Check sheet for the modelled part. Datum: model origin and axes. Units: mm. Face numbers are marked on the shaded views. A direction names the side the tool comes from. Give positions to 0.01 mm unless a question says otherwise; leave off trailing zeros. Order: outer loops, then holes, each group sorted by start corner. A loop starts at its lowest first (then second) coordinate and runs counter-clockwise, first axis right, second up.
from build123d import *

# Parameters (mm, degrees)
F0_R      = 100
F1_DEPTH  = 50
F2_R      = 10
F1_FACE_R = 90
F3_DEPTH  = 3
F5_DEPTH  = 3
F7_W      = 2.681116
F7_H      = 11.75565
F7_W_2    = 14
F7_H_2    = 14
F8_DEPTH  = 3


with BuildPart() as f1:
    # F0 (on Top) → F1 (new body)
    with BuildSketch(Plane.XY):
        Circle(F0_R)
    extrude(amount=F1_DEPTH)

    # F2
    f2_edges = [f1.edges().sort_by_distance(p)[0] for p in [
        (-100, 0, 50),
    ]]
    fillet(f2_edges, radius=F2_R)

    # F1_face (on face) → F3 (cut)
    with BuildSketch(Plane.XY.offset(50)):
        Circle(F1_FACE_R)
    extrude(amount=-F3_DEPTH, mode=Mode.SUBTRACT)

    # F4 (on face) → F5 (join)
    with BuildSketch(Plane.XY.offset(47)):
        with BuildLine():
            ThreePointArc((53.019027, 62.901433), (33.066942, 75.327185), (10.415382, 81.603476))
            ThreePointArc((10.415382, 81.603476), (6.603495, 80.503103), (4.793179, 76.972655))
            Line((4.793179, 76.972655), (0, 4.273428))
            ThreePointArc((0, 4.273428), (1.220514, 4.095428), (2.339353, 3.576257))
            Line((2.339353, 3.576257), (53.365395, 55.576407))
            ThreePointArc((53.365395, 55.576407), (54.791012, 59.31452), (53.019027, 62.901433))
        make_face()
        with BuildLine():
            Line((60.673054, 47.679128), (3.6639, 2.19955))
            ThreePointArc((3.6639, 2.19955), (4.118228, 1.141221), (4.273428, 0))
            Line((4.273428, 0), (77.20216, 0))
            ThreePointArc((77.20216, 0), (80.850155, 1.580624), (82.191706, 5.323148))
            ThreePointArc((82.191706, 5.323148), (77.83869, 26.924909), (67.913987, 46.599387))
            ThreePointArc((67.913987, 46.599387), (64.528614, 48.715836), (60.673054, 47.679128))
        make_face()
        with BuildLine():
            Line((76.89521, -7.459046), (4.048797, -1.367271))
            ThreePointArc((4.048797, -1.367271), (3.521918, -2.420388), (2.727619, -3.289723))
            Line((2.727619, -3.289723), (59.141904, -49.88977))
            ThreePointArc((59.141904, -49.88977), (62.935195, -50.997631), (66.348065, -49.005464))
            ThreePointArc((66.348065, -49.005464), (76.013771, -32.023551), (81.413661, -13.244508))
            ThreePointArc((81.413661, -13.244508), (80.419138, -9.364044), (76.89521, -7.459046))
        make_face()
        with BuildLine():
            Line((53.523655, -55.496099), (1.881672, -3.83686))
            ThreePointArc((1.881672, -3.83686), (0.965826, -4.162855), (0, -4.273428))
            Line((0, -4.273428), (0, -77.190785))
            ThreePointArc((0, -77.190785), (1.580642, -80.838796), (5.323196, -82.180328))
            ThreePointArc((5.323196, -82.180328), (30.825875, -76.365622), (53.21868, -62.846757))
            ThreePointArc((53.21868, -62.846757), (54.983233, -59.238312), (53.523655, -55.496099))
        make_face()
        with BuildLine():
            ThreePointArc((-1.125943, -4.122431), (-1.961033, -3.796911), (-2.709859, -3.304368))
            Line((-2.709859, -3.304368), (-51.280371, -57.962817))
            ThreePointArc((-51.280371, -57.962817), (-52.52156, -61.744691), (-50.6076, -65.234659))
            ThreePointArc((-50.6076, -65.234659), (-33.298804, -75.55051), (-14.006687, -81.366471))
            ThreePointArc((-14.006687, -81.366471), (-10.12515, -80.413756), (-8.181768, -76.921298))
            Line((-8.181768, -76.921298), (-1.125943, -4.122431))
        make_face()
        with BuildLine():
            ThreePointArc((-3.751637, -2.046315), (-4.140926, -1.055896), (-4.273428, 0))
            Line((-4.273428, 0), (-76.929663, 0))
            ThreePointArc((-76.929663, 0), (-80.578049, -1.581041), (-81.919135, -5.324288))
            ThreePointArc((-81.919135, -5.324288), (-76.277786, -30.344556), (-63.190557, -52.402731))
            ThreePointArc((-63.190557, -52.402731), (-59.607242, -54.203971), (-55.85314, -52.792826))
            Line((-55.85314, -52.792826), (-3.751637, -2.046315))
        make_face()
        with BuildLine():
            ThreePointArc((-3.992636, 1.523496), (-3.70279, 2.133433), (-3.320478, 2.690094))
            Line((-3.320478, 2.690094), (-56.699298, 51.911248))
            ThreePointArc((-56.699298, 51.911248), (-60.462161, 53.221499), (-63.987913, 51.365437))
            ThreePointArc((-63.987913, 51.365437), (-75.024742, 33.228741), (-81.038817, 12.867449))
            ThreePointArc((-81.038817, 12.867449), (-80.025089, 8.98514), (-76.484046, 7.098084))
            Line((-76.484046, 7.098084), (-3.992636, 1.523496))
        make_face()
        with BuildLine():
            ThreePointArc((-2.536746, 3.439056), (-1.913037, 3.821319), (-1.233269, 4.091605))
            Line((-1.233269, 4.091605), (-5.433671, 76.419476))
            ThreePointArc((-5.433671, 76.419476), (-7.248956, 79.99108), (-11.103634, 81.083359))
            ThreePointArc((-11.103634, 81.083359), (-32.563457, 75.082775), (-51.60924, 63.516046))
            ThreePointArc((-51.60924, 63.516046), (-53.4449, 59.971321), (-52.100808, 56.212578))
            Line((-52.100808, 56.212578), (-2.536746, 3.439056))
        make_face()
    extrude(amount=F5_DEPTH)

    # F7 (on face) → F8 (join)
    with BuildSketch(Plane.XY.offset(50)):
        Polygon((24.804033, 61.312177), (10.367269, 71.005437), (10.367269, 52.856359), align=None)
        Polygon((35.528484, 62.137136), (7.479916, 45.844217), (8.79458, 43.327766), (36.953135, 59.684574), align=None)
        with Locations((19.957405, 39.966392)):
            Rectangle(F7_W, F7_H)
        with Locations((26.019179, 39.966392)):
            Rectangle(F7_W, F7_H)
        with Locations((-21.684457, -47.305547)):
            Rectangle(F7_W_2, F7_H_2)
        Polygon((42.08035, -15.2739), (32.804038, -10.438373), (32.804038, -20.701531), align=None)
        Polygon((51.35667, -15.2739), (42.27772, -10.438373), (42.27772, -20.898901), align=None)
        Polygon((-49.238652, 19.220938), (-39.96234, 14.385412), (-39.96234, 24.64857), align=None)
        Polygon((-58.514971, 19.220938), (-49.436022, 14.385412), (-49.436022, 24.845939), align=None)
    extrude(amount=F8_DEPTH)


solid = f1.part
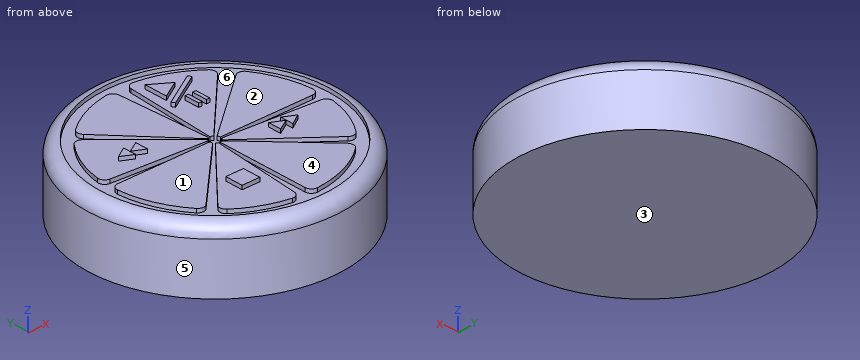
1) Section check A-A, the plane z = 37. Record the cut outline in (x, y), then the cut area to 3 significant figures.
Recorded:
outline: circle Ø200 at (0, 0)
area: 31,400 mm2
2) Material ranges on L1, parallel to Z at x = 61, y = 5; L2, parallel to X at y = 33.5, z = 48.5; L3, parallel to Z at x = 69.5, y = 55, recorded low to high.
Recorded:
L1: z = 0 to 50
L2: x = -89.18 to -83.53, -74.9 to -36.73, -30.77 to -2.94, 1.93 to 31.7, 42.9 to 75.24, 83.53 to 89.18
L3: z = 0 to 47
3) Depth check by flat-ended pin: pin 1 Ø0.9 at (y, z) = (-16, 51) entering from -X; pin 2 Ø0.9 at (y, z) = (63.5, 51) entering from -X; pin 3 Ø1.5 at (x, z) = (-23.5, 51) entering from +Y; pin 4 Ø4 at (x, y) = (56, 79.5) entering from -Z. Enter the tip coordinate at first touch or a pass-through.
Recorded:
pin 1: stops at x = 32.8
pin 2: stops at x = 10.37
pin 3: stops at y = -40.31
pin 4: stops at z = 0
4) Draft check along Y on the marked faces 4, 5 and 6. Enter one of: +Y half, -Y half, draft (parallel to the pull), parting line (faces both ways), or undercut.
Recorded:
face 4: draft
face 5: parting line
face 6: undercut
5) Set-up check for the marked faces 1, 2 and 3: record each of +Z, -Z, +X, -X, +Y, -Y from which the full face is reachable in a straight line by a thin tool's end or side.
Recorded:
face 1: +Z, -X
face 2: +Z, +X
face 3: -Z, +X, -X, +Y, -Y
